from build123d import *

# Parameters (mm, degrees)
SKETCH1_R                = 13.75
SKETCH1_R_2              = 4.15
BOSS_EXTRUDE1_DEPTH      = 2.5
SKETCH2_R                = 6.5
SKETCH2_R_2              = 4.15
BOSS_EXTRUDE2_DEPTH      = 2.5
CUT_EXTRUDE1_DEPTH       = 21.077973005
FILLET1_R                = 0.5
CIRPATTERN1_COUNT        = 4
FILLET1_OF_CIRPATTERN1_R = 0.5


with BuildPart() as part:
    # Sketch1 → Boss-Extrude1 (new body)
    with BuildSketch(Plane.XY):
        Circle(SKETCH1_R)
        Circle(SKETCH1_R_2, mode=Mode.SUBTRACT)
    extrude(amount=BOSS_EXTRUDE1_DEPTH)

    # Sketch2 → Boss-Extrude2 (add)
    with BuildSketch(Plane.XY.offset(2.5)):
        Circle(SKETCH2_R)
        Circle(SKETCH2_R_2, mode=Mode.SUBTRACT)
    extrude(amount=BOSS_EXTRUDE2_DEPTH)

    # Sketch5 → Cut-Extrude1 (cut, through all)
    with BuildSketch(Plane.XY):
        with BuildLine():
            Line((0, 12.75), (0, 7.5))
            ThreePointArc((0, 7.5), (2.870125743, 6.929096494), (5.303300859, 5.303300859))
            Line((5.303300859, 5.303300859), (9.01561146, 9.01561146))
            ThreePointArc((9.01561146, 9.01561146), (4.879213763, 11.77946404), (0, 12.75))
        make_face()
    cut_extrude1 = extrude(amount=CUT_EXTRUDE1_DEPTH, mode=Mode.SUBTRACT)

    # Fillet1
    fillet1_edges = [part.edges().sort_by_distance(p)[0] for p in [
        (0, 7.5, 1.25),
        (5.303300859, 5.303300859, 1.25),
        (9.01561146, 9.01561146, 1.25),
        (0, 12.75, 1.25),
    ]]
    fillet(fillet1_edges, radius=FILLET1_R)

    # CirPattern1: Cut-Extrude1 ×4 about axis
    cirpattern1_axis = Axis((0, 0, 0), (0, 0, 1))
    for i in range(1, CIRPATTERN1_COUNT):
        add(cut_extrude1.rotate(cirpattern1_axis, i * 360 / CIRPATTERN1_COUNT), mode=Mode.SUBTRACT)

    # Fillet1 of CirPattern1
    fillet1_of_cirpattern1_edges = [part.edges().sort_by_distance(p)[0] for p in [
        (-7.5, 0, 1.25),
        (-5.303300859, 5.303300859, 1.25),
        (-9.01561146, 9.01561146, 1.25),
        (-12.75, 0, 1.25),
        (0, -7.5, 1.25),
        (-5.303300859, -5.303300859, 1.25),
        (-9.01561146, -9.01561146, 1.25),
        (0, -12.75, 1.25),
        (7.5, 0, 1.25),
        (5.303300859, -5.303300859, 1.25),
        (9.01561146, -9.01561146, 1.25),
        (12.75, 0, 1.25),
    ]]
    fillet(fillet1_of_cirpattern1_edges, radius=FILLET1_OF_CIRPATTERN1_R)


solid = part.part
For this review, take the finished solid that the model builds, in its own axes (mm). A direction names the side the tool comes from. Coordinates: 2 decimals unless noted, no trailing zeros. Loops run counter-clockwise (first coordinate to the right, second up) from the corner with the lowest first, then second, coordinate; pieces in that order, holes last. Notation, with made-up numbers: (34, 76) - (38, 76) arc R24 cw to (38, 112) - close; hole circle Ø6 at (46.5, 21.25). An arc over 180 degrees is marked (long way). Return JSON: item names as keys, results as strings.
Item 1: For faces 5 (the cylindrical face through (4.937, 11.755, 1.232)), 6 (the flat face through (1.4, -4.2, 5)), list the 3-axis set-ups (+Z, -Z, +X, -X, +Y, -Y) from which the entire face can be reached by the end or side of a thin tool; tool diameter is ignored.
Determined:
{"face 5": "+Z, -Z", "face 6": "+Z, +X, -X, +Y, -Y"}
Item 2: Mouldability with a two-part tool opening along Y and no side actions: class faces 1 (the flat face through (-7, -7, 1)), 2 (the cylindrical face through (2.84, 6.94, 1.23)), 3 (the cylindrical face through (-5.158, -3.955, 3.732)), 4 (the flat face through (6, -3, 2.5)) as pulls with the +Y half, pulls with the -Y half, needs draft (parallel to the pull), parting line crosses it, or undercut.
Determined:
{"face 1": "undercut", "face 2": "undercut", "face 3": "parting line crosses it", "face 4": "needs draft"}
Item 3: For line 1 (X direction, y = 6.75, z = 0.7); line 2 (Y direction, x = 0, z = 3.85); line 3 (X direction, y = 2, z = 0.85), list the stretches that pass through material, from the lowest coordinate up.
Determined:
{"line 1": "x = -11.98 to -10.82, -6.75 to 3.27, 6.75 to 11.98", "line 2": "y = -6.5 to -4.15, 4.15 to 6.5", "line 3": "x = -13.6 to -12.59, -7.23 to -3.64, 3.64 to 13.6"}
Item 4: Take a section at A-A (x = 7). Give the boundary of the cut face in (y, z).
Determined:
{"outline": "(-11.83, 0) - (-7, 0) - (-7, 2.5) - (-11.83, 2.5) - close; (-2.69, 0) - (7, 0) - (7, 2.5) - (-2.69, 2.5) - close; (10.66, 0) - (11.83, 0) - (11.83, 2.5) - (10.66, 2.5) - close"}
Item 5: Take a section at B-B (z = 3.4). Give the boundary of the cut face in (x, y), then the cut area to 3 significant figures.
Determined:
{"outline": "circle Ø13 at (0, 0); hole circle Ø8.3 at (0, 0)", "area": "78.6 mm2"}
Item 6: Insertion check: pin 1 (3 mm diameter, centred on x = 11, z = 1, fed in from -Y); pin 2 (1.5 mm diameter, centred on x = 10.5, y = 1, fed in from +Z); pin 3 (1 mm diameter, centred on x = 8.5, y = -7, fed in from +Z); pin 4 (0.8 mm diameter, centred on x = -10.5, z = 1.5, fed in from +Y). Each pin has a flat end and moves straight along its axis. Give the tip position at first contact, or say it passes through.
Determined:
{"pin 1": "stops at y = -9.94", "pin 2": "stops at z = 2.5", "pin 3": "passes through", "pin 4": "stops at y = 9.33"}
